The model under review builds one solid part; all positions refer to its coordinate system, in mm. A direction names the side the tool comes from. Coordinates: 2 decimals unless noted, no trailing zeros. Order: outer loops, then holes, each group sorted by start corner. A loop starts at its lowest first (then second) coordinate and runs counter-clockwise, first axis right, second up.
```python
from build123d import *

# Parameters (mm, degrees)
SKETCH_1_R          = 30
EXTRUDE_1_DEPTH     = 5
SKETCH_3_R          = 2.75
CUT_EXTRUDE_2_DEPTH = 20
SKETCH_4_R          = 2.75
CUT_EXTRUDE_3_DEPTH = 10
SKETCH_10_W         = 76
SKETCH_10_H         = 34.93
SKETCH_10_R         = 2.5
SKETCH_10_R_2       = 2.75
EXTRUDE_2_DEPTH     = 5


with BuildPart() as part:
    # 草图1 → 凸台-拉伸1 (new body)
    with BuildSketch(Plane.XY):
        with BuildLine():
            Line((-48, 109.07), (-48, 0))
            Line((-48, 0), (48, 0))
            Line((48, 0), (48, 109.07))
            ThreePointArc((48, 109.07), (0, 145.07), (-48, 109.07))
        make_face()
        with Locations((0, 95.07)):
            Circle(SKETCH_1_R, mode=Mode.SUBTRACT)
    extrude(amount=EXTRUDE_1_DEPTH)

    # 草图3 → 切除-拉伸2 (cut)
    with BuildSketch(Plane.XY.offset(5)):
        with Locations((0, 40)):
            Circle(SKETCH_3_R)
    extrude(amount=-CUT_EXTRUDE_2_DEPTH, mode=Mode.SUBTRACT)

    # 草图4 → 切除-拉伸3 (cut)
    with BuildSketch(Plane.XY.offset(5)):
        with Locations((9.058666579, 128.87740392)):
            Circle(SKETCH_4_R)
        with Locations((24.748737342, 119.818737342)):
            Circle(SKETCH_4_R)
        with Locations((33.80740392, 104.128666579)):
            Circle(SKETCH_4_R)
        with Locations((33.80740392, 86.011333421)):
            Circle(SKETCH_4_R)
        with Locations((24.748737342, 70.321262658)):
            Circle(SKETCH_4_R)
        with Locations((9.058666579, 61.26259608)):
            Circle(SKETCH_4_R)
        with Locations((-9.058666579, 61.26259608)):
            Circle(SKETCH_4_R)
        with Locations((-24.748737342, 70.321262658)):
            Circle(SKETCH_4_R)
        with Locations((-33.80740392, 86.011333421)):
            Circle(SKETCH_4_R)
        with Locations((-33.80740392, 104.128666579)):
            Circle(SKETCH_4_R)
        with Locations((-24.748737342, 119.818737342)):
            Circle(SKETCH_4_R)
        with Locations((-9.058666579, 128.87740392)):
            Circle(SKETCH_4_R)
    extrude(amount=-CUT_EXTRUDE_3_DEPTH, mode=Mode.SUBTRACT)

    # 草图10 → 凸台-拉伸2 (add)
    with BuildSketch(Plane.XY.offset(5)):
        with Locations((0, -17.465)):
            Rectangle(SKETCH_10_W, SKETCH_10_H)
        with Locations((25, -14.93)):
            Circle(SKETCH_10_R, mode=Mode.SUBTRACT)
        with Locations((-25, -14.93)):
            Circle(SKETCH_10_R, mode=Mode.SUBTRACT)
        with Locations((0, -14.93)):
            Circle(SKETCH_10_R_2, mode=Mode.SUBTRACT)
    extrude(amount=-EXTRUDE_2_DEPTH)


solid = part.part
```
(1) We need section D-D, the plane x = -16. Write out the cut boundary in (y, z).
A:
outline: (-34.93, 0) - (69.69, 0) - (69.69, 5) - (-34.93, 5) - close; (120.45, 0) - (142.44, 0) - (142.44, 5) - (120.45, 5) - close
(2) Wall thickness on probe 1 along Y at (x, z) = (-9, 4); probe 2 along Y at (x, z) = (2.5, 2); probe 3 along X at (y, z) = (69, 0.65): over which ranges is each line inside the solid? List them lowest first.
A:
probe 1: y = -34.93 to 58.51, 64.01 to 66.45, 123.69 to 126.13, 131.63 to 144.25
probe 2: y = -34.93 to -16.08, -13.78 to 38.85, 41.15 to 65.17, 124.97 to 145.01
probe 3: x = -48 to -27.16, -22.34 to -14.84, 14.84 to 22.34, 27.16 to 48
(3) For pin 1 Ø12 at (x, y) = (27, 120) entering from -Z; pin 2 Ø1 at (y, z) = (-7.5, 3) entering from -X; pin 3 Ø2.5 at (x, z) = (42.5, 1.5) entering from -Y, all flat-tipped, find the tip position at first contact; note any pin that passes through.
A:
pin 1: stops at z = 0
pin 2: stops at x = -38
pin 3: stops at y = 0
(4) Draft analysis for pull direction Y (two halves, no side actions). For faces 1 (the face through (-38, -18, 3)), 2 (the face through (-34.404, 83.327, 2.535)), 3 (the face through (43, 0, 2)), state which applies: released by +Y, released by -Y, zero draft, split by the parting line, or undercut.
A:
face 1: zero draft
face 2: undercut
face 3: released by -Y
(5) Machinability: for faces 4 (the face through (38, -18, 3)), 5 (the face through (-1, -34.93, 3)), which of the approach directions +Z, -Z, +X, -X, +Y, -Y give a long, thin tool a straight path to every point of the face, cutting with its end or side? Answer none if there is none.
A:
face 4: +Z, -Z, +X, -Y
face 5: +Z, -Z, +X, -X, -Y
(6) We need section A-A, the plane x = 0. Write out the cut boundary in (y, z).
A:
outline: (-34.93, 0) - (-17.68, 0) - (-17.68, 5) - (-34.93, 5) - close; (-12.18, 0) - (37.25, 0) - (37.25, 5) - (-12.18, 5) - close; (42.75, 0) - (65.07, 0) - (65.07, 5) - (42.75, 5) - close; (125.07, 0) - (145.07, 0) - (145.07, 5) - (125.07, 5) - close
(7) We need section C-C, the plane y = 95.07. Write out the cut boundary in (x, z), and give its area (3 significant figures).
A:
outline: (-48, 0) - (-30, 0) - (-30, 5) - (-48, 5) - close; (30, 0) - (48, 0) - (48, 5) - (30, 5) - close
area: 180 mm2
(8) We need section B-B, the plane y = -14.93. Write out the cut boundary in (x, z), and give its area (4 significant figures).
A:
outline: (-38, 0) - (-27.5, 0) - (-27.5, 5) - (-38, 5) - close; (-22.5, 0) - (-2.75, 0) - (-2.75, 5) - (-22.5, 5) - close; (2.75, 0) - (22.5, 0) - (22.5, 5) - (2.75, 5) - close; (27.5, 0) - (38, 0) - (38, 5) - (27.5, 5) - close
area: 302.5 mm2
